Part model, mm, in its own coordinate system. A direction names the side the tool comes from. Give positions to 0.01 mm unless a question says otherwise; leave off trailing zeros. Order: outer loops, then holes, each group sorted by start corner. A loop starts at its lowest first (then second) coordinate and runs counter-clockwise, first axis right, second up. Notation, with made-up numbers: M 10.5,43 L 63.5,43 A17 cw 63.5,69 Z; hole C -14,33 d2. An arc over 180 degrees is marked long. Return JSON: item names as keys, results as strings.
from build123d import *

# Parameters (mm, degrees)
F1_DEPTH = 3.81
F2_DEPTH = 11.43
F3_DEPTH = 1.905
F4_DEPTH = 0.635
F5_DEPTH = 0.381


with BuildPart() as f1:
    # F0 (on Top) → F1 (new body)
    with BuildSketch(Plane.XY):
        with BuildLine():
            Line((0, 40.64), (0, 20.32))
            Line((0, 20.32), (36.0270839263, 46.3555857197))
            ThreePointArc((36.0270839263, 46.3555857197), (32.7743226286, 46.8899395332), (29.8984857282, 48.5010112824))
            ThreePointArc((29.8984857282, 48.5010112824), (28.8184538619, 49.5338980727), (27.9132711745, 50.7230020447))
            ThreePointArc((27.9132711745, 50.7230020447), (26.7835232138, 53.1922797151), (26.3964543073, 55.88))
            Line((26.3964543073, 55.88), (0, 40.64))
        make_face()
        with BuildLine():
            Line((0, 20.32), (0, 0))
            Line((0, 0), (30.7958633586, -17.78))
            ThreePointArc((30.7958633586, -17.78), (29.7012441826, -13.6075167511), (30.5594271825, -9.3800672195))
            ThreePointArc((30.5594271825, -9.3800672195), (31.4801291394, -7.7913902048), (32.6885555919, -6.4088952646))
            ThreePointArc((32.6885555919, -6.4088952646), (38.1196995449, -3.8785721663), (43.9872077535, -5.0919175595))
            Line((43.9872077535, -5.0919175595), (0, 20.32))
        make_face()
        with BuildLine():
            Line((-54.9258633586, -17.78), (-24.13, 0))
            Line((-24.13, 0), (-24.13, 20.32))
            Line((-24.13, 20.32), (-68.1172077535, -5.0919175595))
            ThreePointArc((-68.1172077535, -5.0919175595), (-62.2496995449, -3.8785721663), (-56.8185555919, -6.4088952646))
            ThreePointArc((-56.8185555919, -6.4088952646), (-55.6101291394, -7.7913902048), (-54.6894271825, -9.3800672195))
            ThreePointArc((-54.6894271825, -9.3800672195), (-54.0454560084, -11.3134252867), (-53.8274732111, -13.3395190133))
            ThreePointArc((-53.8274732111, -13.3395190133), (-54.1061473504, -15.6266751246), (-54.9258633586, -17.78))
        make_face()
        with BuildLine():
            Line((-66.0401488201, 49.028525317), (-24.13, 20.32))
            Line((-24.13, 20.32), (-24.13, 40.64))
            Line((-24.13, 40.64), (-54.9258633586, 58.42))
            ThreePointArc((-54.9258633586, 58.42), (-55.2263237646, 56.0465016792), (-56.1087492964, 53.8227445173))
            ThreePointArc((-56.1087492964, 53.8227445173), (-57.3142816625, 52.1116859071), (-58.8644308605, 50.7052480957))
            ThreePointArc((-58.8644308605, 50.7052480957), (-62.2835733625, 49.1448461429), (-66.0401488201, 49.028525317))
        make_face()
        Polygon((-24.13, 0), (0, 0), (0, 20.32), (0, 40.64), (-24.13, 40.64), (-24.13, 20.32), align=None)
        Polygon((-18.3272082359, 2.3950056639), (-21.7771697789, 2.3950056639), (-21.7771697789, 5.8912090026), (-21.7771697789, 34.7188413143), (-21.7771697789, 39.2318554223), (-18.1576330215, 39.2318554223), (-4.7612613998, 39.2318554223), (-1.5657880576, 39.2318554223), (-1.5657880576, 35.2370127553), (-1.5657880576, 6.7390808836), (-1.5657880576, 2.3950056639), (-5.2699861117, 2.3950056639), align=None, mode=Mode.SUBTRACT)
    extrude(amount=F1_DEPTH)

    # F0 (on Top) → F2 (join)
    with BuildSketch(Plane.XY):
        with BuildLine():
            ThreePointArc((30.5594271825, -9.3800672195), (29.7012441826, -13.6075167511), (30.7958633586, -17.78))
            ThreePointArc((30.7958633586, -17.78), (41.5096293224, -22.585844874), (48.7474732111, -13.3395190133))
            ThreePointArc((48.7474732111, -13.3395190133), (47.4720102137, -8.5781364156), (43.9872077535, -5.0919175595))
            ThreePointArc((43.9872077535, -5.0919175595), (38.1196995449, -3.8785721663), (32.6885555919, -6.4088952646))
            Line((32.6885555919, -6.4088952646), (36.5475066082, -9.0208440228))
            ThreePointArc((36.5475066082, -9.0208440228), (41.6940688149, -8.9013194717), (44.3024732111, -13.3395190133))
            ThreePointArc((44.3024732111, -13.3395190133), (38.3505482132, -18.3441315655), (34.4417854953, -11.6215478365))
            Line((34.4417854953, -11.6215478365), (30.5594271825, -9.3800672195))
        make_face()
        with BuildLine():
            ThreePointArc((-68.1172077535, -5.0919175595), (-69.9554416118, -20.2043885167), (-54.9258633586, -17.78))
            ThreePointArc((-54.9258633586, -17.78), (-54.1061473504, -15.6266751246), (-53.8274732111, -13.3395190133))
            ThreePointArc((-53.8274732111, -13.3395190133), (-54.0454560084, -11.3134252867), (-54.6894271825, -9.3800672195))
            Line((-54.6894271825, -9.3800672195), (-58.5717854953, -11.6215478365))
            ThreePointArc((-58.5717854953, -11.6215478365), (-58.3478606589, -12.4675940154), (-58.2724732111, -13.3395190133))
            ThreePointArc((-58.2724732111, -13.3395190133), (-67.7906727527, -15.8111146171), (-60.6775066082, -9.0208440228))
            Line((-60.6775066082, -9.0208440228), (-56.8185555919, -6.4088952646))
            ThreePointArc((-56.8185555919, -6.4088952646), (-62.2496995449, -3.8785721663), (-68.1172077535, -5.0919175595))
        make_face()
        with BuildLine():
            ThreePointArc((-54.9258633586, 58.42), (-70.5985328755, 65.6954233217), (-66.0401488201, 49.028525317))
            ThreePointArc((-66.0401488201, 49.028525317), (-62.2835733625, 49.1448461429), (-58.8644308605, 50.7052480957))
            Line((-58.8644308605, 50.7052480957), (-62.5780124602, 53.6978363526))
            ThreePointArc((-62.5780124602, 53.6978363526), (-68.6532723441, 61.2741476343), (-59.3708633586, 58.42))
            ThreePointArc((-59.3708633586, 58.42), (-59.5311595199, 57.153937545), (-60.0019319176, 55.9677746772))
            Line((-60.0019319176, 55.9677746772), (-56.1087492964, 53.8227445173))
            ThreePointArc((-56.1087492964, 53.8227445173), (-55.2263237646, 56.0465016792), (-54.9258633586, 58.42))
        make_face()
        with BuildLine():
            ThreePointArc((29.8984857282, 48.5010112824), (32.7743226286, 46.8899395332), (36.0270839263, 46.3555857197))
            ThreePointArc((36.0270839263, 46.3555857197), (42.6938891398, 49.1822577357), (45.4464543073, 55.88))
            ThreePointArc((45.4464543073, 55.88), (35.9214543073, 65.405), (26.3964543073, 55.88))
            ThreePointArc((26.3964543073, 55.88), (26.7835232138, 53.1922797151), (27.9132711745, 50.7230020447))
            Line((27.9132711745, 50.7230020447), (31.5300523665, 53.3261814877))
            ThreePointArc((31.5300523665, 53.3261814877), (34.598941899, 60.7848303671), (41.0014543073, 55.88))
            ThreePointArc((41.0014543073, 55.88), (38.820808345, 51.708651757), (34.1510030615, 51.1184978855))
            Line((34.1510030615, 51.1184978855), (29.8984857282, 48.5010112824))
        make_face()
    extrude(amount=F2_DEPTH)

    # F0 (on Top) → F3 (join)
    with BuildSketch(Plane.XY):
        Polygon((-21.7771697789, 5.8912090026), (-21.7771697789, 2.3950056639), (-18.3272082359, 2.3950056639), (-16.8476979102, 5.2939299848), (-21.0003481494, 7.4132984911), align=None)
        Polygon((-6.7851137214, 5.3618797736), (-5.2699861117, 2.3950056639), (-1.5657880576, 2.3950056639), (-1.5657880576, 6.7390808836), (-2.0874397167, 7.760661653), align=None)
        Polygon((-21.7771697789, 39.2318554223), (-21.7771697789, 34.7188413143), (-20.8961134896, 32.993585252), (-16.1974461672, 35.3931075525), (-18.1576330215, 39.2318554223), align=None)
        Polygon((-2.074527, 34.2401993722), (-1.5657880576, 35.2370127553), (-1.5657880576, 39.2318554223), (-4.7612613998, 39.2318554223), (-6.2271772392, 36.3595678785), align=None)
    extrude(amount=F3_DEPTH)

    # F0 (on Top) → F4 (join)
    with BuildSketch(Plane.XY):
        Polygon((-21.0003481494, 7.4132984911), (-16.8476979102, 5.2939299848), (-11.8006188508, 15.1830804564), (-6.7851137214, 5.3618797736), (-2.0874397167, 7.760661653), (-8.8398640982, 20.9843268631), (-2.074527, 34.2401993722), (-6.2271772392, 36.3595678785), (-11.4576985252, 26.110984206), (-16.1974461672, 35.3931075525), (-20.8961134896, 32.993585252), (-14.41858046, 20.309488601), align=None)
    extrude(amount=F4_DEPTH)

    # F0 (on Top) → F5 (join)
    with BuildSketch(Plane.XY):
        with BuildLine():
            Line((-24.13, 40.64), (0, 40.64))
            ThreePointArc((0, 40.64), (-12.065, 49.8591743067), (-24.13, 40.64))
        make_face()
    extrude(amount=F5_DEPTH)


solid = f1.part
Q1. Band-saw the part on C-C (y = 38). Give the cut face in (x, z) (3 decimals).
Established:
{"outline": "M -49.94,0 L -17.529,0 L -17.529,1.905 L -21.777,1.905 L -21.777,3.81 L -49.94,3.81 Z; M -5.39,0 L 24.465,0 L 24.465,3.81 L -1.566,3.81 L -1.566,1.905 L -5.39,1.905 Z"}
Q2. Band-saw the part on B-B (x = -38.5). Give the cut face in (y, z).
Established:
{"outline": "M -8.3,0 L 12.02,0 L 12.02,3.81 L -8.3,3.81 Z; M 30.16,0 L 48.94,0 L 48.94,3.81 L 30.16,3.81 Z"}
Q3. Pin check, flat tips, straight feed: pin 1 (1.9 mm diameter, centred on y = 29.5, z = 2.5, fed in from -X); pin 2 (1.5 mm diameter, centred on x = 6.5, z = 4, fed in from -Y); pin 3 (1.1 mm diameter, centred on x = -13, z = 2.5, fed in from -Y). Stop position of each tip, or through.
Established:
{"pin 1": "stops at x = -38.92", "pin 2": "stops at y = -4.17", "pin 3": "stops at y = 0"}
Q4. Band-saw the part on A-A (z = 5.75). Give the number of separate pieces and of enclosed holes in the cut face, then the cut area to 3 significant figures.
Established:
{"separate pieces": "4", "enclosed holes": "0", "area": "753 mm²"}
Q5. Two-plate mould, pull along Y, no slides. Class faces 1 (the flat face through (-12, 44, 0.381)), 2 (the flat face through (-12, 0, 2)), 3 (the flat face through (13.383, 48.367, 1.878)), 4 (the cylindrical face through (-57.295, 52.134, 1.878)): +Y half, -Y half, draft (parallel to the pull), parting line (faces both ways), or undercut.
Established:
{"face 1": "draft", "face 2": "-Y half", "face 3": "+Y half", "face 4": "undercut"}
Q6. Probe line 1 along X through (y, z) = (55.88, 4.5); line 2 along Y through (x, z) = (39, 7); line 3 along Y through (x, z) = (-58, 8.5). List the from-to ranges inside material, lowest first.
Established:
{"line 1": "x = -73.63 to -68.85, -59.84 to -55.27, 26.4 to 30.84, 41 to 45.45", "line 2": "y = -22.86 to -18.41, -8.26 to -3.82, 46.87 to 51.84, 59.92 to 64.89", "line 3": "y = -21.22 to -11.29, -7.21 to -5.46, 54.86 to 65.43"}
Q7. 3-axis set-ups, long thin cutter, end or side, ignore diameter. For faces 5 (the flat face through (22.302, 7.436, 1.878)), 6 (the flat face through (-12, 40.64, 2)), 7 (the flat face through (-4, 5, 1.905)), 8 (the flat face through (-39.3, 49.4, 1.9)): which of +Z, -Z, +X, -X, +Y, -Y reach the whole face in a straight line?
Established:
{"face 5": "+Z, -Z, +X", "face 6": "+Z, +Y", "face 7": "+Z", "face 8": "+Z, -Z, +Y"}
